from build123d import *

# Parameters (mm, degrees)
F1_DEPTH       = 6
F2_D           = 5.5
F2_DEPTH       = 19
F2_CSINK_D     = 11.2
F2_CSINK_ANGLE = 90
F2_TIP         = 1.6523667023
F4_D           = 3.3
F4_DEPTH       = 14.1
F4_TIP         = 0.9914200214


with BuildPart() as f1:
    # F0 (on Front) → F1 (new body)
    with BuildSketch(Plane.XZ):
        with BuildLine():
            Line((28, 40), (-28, 40))
            ThreePointArc((-28, 40), (-29.4142135624, 39.4142135624), (-30, 38))
            Line((-30, 38), (-30, -38))
            ThreePointArc((-30, -38), (-29.4142135624, -39.4142135624), (-28, -40))
            Line((-28, -40), (28, -40))
            ThreePointArc((28, -40), (29.4142135624, -39.4142135624), (30, -38))
            Line((30, -38), (30, 38))
            ThreePointArc((30, 38), (29.4142135624, 39.4142135624), (28, 40))
        make_face()
        with BuildLine():
            Line((-16, -23), (-16, 31))
            ThreePointArc((-16, 31), (-15.1213203436, 33.1213203436), (-13, 34))
            ThreePointArc((-13, 34), (-10.8786796564, 33.1213203436), (-10, 31))
            Line((-10, 31), (-10, -23))
            ThreePointArc((-10, -23), (-10.8786796564, -25.1213203436), (-13, -26))
            ThreePointArc((-13, -26), (-15.1213203436, -25.1213203436), (-16, -23))
        make_face(mode=Mode.SUBTRACT)
        with BuildLine():
            Line((10, -23), (10, 31))
            ThreePointArc((10, 31), (10.8786796564, 33.1213203436), (13, 34))
            ThreePointArc((13, 34), (15.1213203436, 33.1213203436), (16, 31))
            Line((16, 31), (16, -23))
            ThreePointArc((16, -23), (15.1213203436, -25.1213203436), (13, -26))
            ThreePointArc((13, -26), (10.8786796564, -25.1213203436), (10, -23))
        make_face(mode=Mode.SUBTRACT)
    extrude(amount=F1_DEPTH)

    # F2
    with Locations(Plane(origin=(0, 0, 0), x_dir=(1, 0, 0), z_dir=(0, 1, 0))):
        with Locations((-20, 32), (20, 32)):
            CounterSinkHole(F2_D / 2, F2_CSINK_D / 2, depth=F2_DEPTH, counter_sink_angle=F2_CSINK_ANGLE)
            with Locations((0, 0, -(F2_DEPTH + F2_TIP / 2))):  # 118° drill point
                Cone(0, F2_D / 2, F2_TIP, mode=Mode.SUBTRACT)

    # F4
    with Locations(Plane.XY.offset(40)):
        with Locations((0, -3)):
            Hole(F4_D / 2, depth=F4_DEPTH)
            with Locations((0, 0, -(F4_DEPTH + F4_TIP / 2))):  # 118° drill point
                Cone(0, F4_D / 2, F4_TIP, mode=Mode.SUBTRACT)


solid = f1.part
Geometry: final body of the model. Coordinates: model frame, mm. A direction names the side the tool comes from. Coordinates: 2 decimals unless noted, no trailing zeros. Loops run counter-clockwise (first coordinate to the right, second up) from the corner with the lowest first, then second, coordinate; pieces in that order, holes last. Notation, with made-up numbers: (16.5, 38.5) - (20.5, 38.5) arc R14 cw to (20.5, 61.5) - close; hole circle Ø7 at (-35.5, 67). An arc over 180 degrees is marked (long way). One line per question, with ' | ' between items. Start each with the question number.
(1) Cut plane B-B on x = -20. Output: boundary loops of the cut face in (y, z), and give its area (3 significant figures).
(2) Reachability of faces 5 (the cylindrical face through (1.31, -4, 32.85)), 6 (the flat face through (16, -3, 4)), 7 (the conical face through (-19.37, -2.71, -29.18)) from +Z, -Z, +X, -X, +Y, -Y: full face, straight path, thin tool, end or side. Return the list, or none.
(3) Cut plane C-C on z = -32. Output: boundary loops of the cut face in (x, y).
(4) Cut plane A-A on z = 10.5. Output: boundary loops of the cut face in (x, y).
(5) Ray query, L1, parallel to X at y = -2.1, z = -10; L2, parallel to X at y = -4.1, z = -32; L3, parallel to Y at x = 0, z = 35.75. Return the intervals inside material, ascending. Write a range as from..to.
(6) First-contact query: pin 1 (2.5 mm diameter, centred on x = 0, y = -3, fed in from +Z); pin 2 (6.5 mm diameter, centred on x = -20, z = -32, fed in from +Y); pin 3 (7 mm diameter, centred on x = 20, z = -32, fed in from +Y). Flat tips, straight axial feed; report the tip coordinate or a pass-through.
(7) Draft query along Z for faces 1 (the cylindrical face through (-19.642, -4.447, -34.727)), 2 (the conical face through (22.29, -2.71, -30.24)), 3 (the flat face through (30, -3, -1)), 4 (the flat face through (0, -1, 40)). Return one class per face: +Z half, -Z half, draft (parallel to the pull), parting line (faces both ways), or undercut.
Here are the results:
1) outline: (-6, -40) - (0, -40) - (0, -37.6) - (-2.85, -34.75) - (-6, -34.75) - close; (-6, -29.25) - (-2.85, -29.25) - (0, -26.4) - (0, 40) - (-6, 40) - close | area: 439 mm²
2) face 5: +Z | face 6: +Y, -Y | face 7: +Y
3) outline: (-30, -6) - (-22.75, -6) - (-22.75, -2.85) - (-25.6, 0) - (-30, 0) - close; (-17.25, -6) - (17.25, -6) - (17.25, -2.85) - (14.4, 0) - (-14.4, 0) - (-17.25, -2.85) - close; (22.75, -6) - (30, -6) - (30, 0) - (25.6, 0) - (22.75, -2.85) - close
4) outline: (-30, -6) - (-16, -6) - (-16, 0) - (-30, 0) - close; (-10, -6) - (10, -6) - (10, 0) - (-10, 0) - close; (16, -6) - (30, -6) - (30, 0) - (16, 0) - close
5) L1: -30..-16, -10..10, 16..30 | L2: -30..-22.75, -17.25..17.25, 22.75..30 | L3: -6..-4.65, -1.35..0
6) pin 1: z = 25.66 | pin 2: y = -2.35 | pin 3: y = -2.1
7) face 1: undercut | face 2: undercut | face 3: draft | face 4: +Z half
